For this review, take the finished solid that the model builds, in its own axes (mm). Round coordinates to 2 decimals unless told otherwise and drop trailing zeros. Order: outer loops, then holes, each group sorted by start corner. A loop starts at its lowest first (then second) coordinate and runs counter-clockwise, first axis right, second up. Notation, with made-up numbers: M 78.25,58 L 114.25,58 A17 ccw 114.25,89 Z; hole C 61,-35 d11. An arc over 180 degrees is marked long. Answer in a Markdown table with one row per item. Add a question column.
```python
from build123d import *

# Parameters (mm, degrees)
SKETCH1_R      = 7.9375
SKETCH1_R_2    = 3.571875
EXTRUDE1_DEPTH = 1.651
FILLET1_R      = 0.254


with BuildPart() as part:
    # Sketch1 → Extrude1 (new body)
    with BuildSketch(Plane(origin=(0, 0, 0), x_dir=(1, 0, 0), z_dir=(0, 1, 0))):
        with Locations(Location((0, 0, 0), (0, 0, 270))):  # turned: the seam where the file's is
            Circle(SKETCH1_R)
        with Locations(Location((0, 0, 0), (0, 0, 270))):  # turned: the seam where the file's is
            Circle(SKETCH1_R_2, mode=Mode.SUBTRACT)
    extrude(amount=EXTRUDE1_DEPTH)

    # Fillet1
    fillet1_edges = [part.edges().sort_by_distance(p)[0] for p in [
        (0, 0, -7.9375),
        (0, 1.651, -7.9375),
        (0, 0, -3.571875),
        (0, 1.651, -3.571875),
    ]]
    fillet(fillet1_edges, radius=FILLET1_R)


solid = part.part
```
1. The part is to be moulded in two halves that separate along Z. For faces 1 (the cylindrical face through (0.16, 0.82, -3.57)), 2 (the flat face through (-2, 0, -4)), 3 (the cylindrical face through (-7.75, 0.82, -1.72)), say which applies: pulls with the +Z half, pulls with the -Z half, needs draft (parallel to the pull), parting line crosses it, or undercut.
2. Consider section A-A on x = 0. Write out the cut boundary in (y, z).
3. Consider section B-B on z = 0. Write out the cut boundary in (x, y), plus the area to 3 significant figures.
4. To check wall thickness, follow probe 1 along X at (y, z) = (0.9, 0); probe 2 along Z at (x, y) = (1.5, 0.8); probe 3 along X at (y, z) = (0.95, 1). State the ranges of each line that lie inside material, in increasing order. Write a range as [from, to].
Solved:
| question | item | result |
|---|---|---|
| 1 | face 1 | undercut |
| 1 | face 2 | needs draft |
| 1 | face 3 | parting line crosses it |
| 2 | outline | M 0,-7.68 A0.25 ccw 0.25,-7.94 L 1.4,-7.94 A0.25 ccw 1.65,-7.68 L 1.65,-3.83 A0.25 ccw 1.4,-3.57 L 0.25,-3.57 A0.25 ccw 0,-3.83 Z; M 0,3.83 A0.25 ccw 0.25,3.57 L 1.4,3.57 A0.25 ccw 1.65,3.83 L 1.65,7.68 A0.25 ccw 1.4,7.94 L 0.25,7.94 A0.25 ccw 0,7.68 Z |
| 3 | outline | M -7.94,0.25 A0.25 ccw -7.68,0 L -3.83,0 A0.25 ccw -3.57,0.25 L -3.57,1.4 A0.25 ccw -3.83,1.65 L -7.68,1.65 A0.25 ccw -7.94,1.4 Z; M 3.57,0.25 A0.25 ccw 3.83,0 L 7.68,0 A0.25 ccw 7.94,0.25 L 7.94,1.4 A0.25 ccw 7.68,1.65 L 3.83,1.65 A0.25 ccw 3.57,1.4 Z |
| 3 | area | 14.3 mm^2 |
| 4 | probe 1 | x = [-7.94, -3.57], [3.57, 7.94] |
| 4 | probe 2 | z = [-7.79, -3.24], [3.24, 7.79] |
| 4 | probe 3 | x = [-7.87, -3.43], [3.43, 7.87] |
